Verification items for the finished model (mm, model axes). Face numbers are marked on the shaded views. Coordinates: 2 decimals unless noted, no trailing zeros. Write each loop counter-clockwise with the first axis right and the second up, starting at its lowest first coordinate (ties: lowest second). Pieces come first, ordered by that corner, then holes.
```python
from build123d import *

# Parameters (mm, degrees)
BOSS_EXTRUDE1_DEPTH = 25.5
SKETCH2_R           = 1.7
CUT_EXTRUDE1_DEPTH  = 31.42466105
FILLET1_R           = 3
SKETCH4_R           = 2.85
CUT_EXTRUDE2_DEPTH  = 30.815096847


with BuildPart() as part:
    # Sketch1 → Boss-Extrude1 (new body)
    with BuildSketch(Plane(origin=(0, 0, 0), x_dir=(0, 0, -1), z_dir=(1, 0, 0))):
        with BuildLine():
            Line((4.080441153, -0.4), (15, -0.4))
            Line((15, -0.4), (15, -3.4))
            Line((15, -3.4), (6.232976817, -3.4))
            ThreePointArc((6.232976817, -3.4), (0, -7.1), (-6.232976817, -3.4))
            Line((-6.232976817, -3.4), (-15, -3.4))
            Line((-15, -3.4), (-15, -0.4))
            Line((-15, -0.4), (-4.080441153, -0.4))
            ThreePointArc((-4.080441153, -0.4), (0, -4.1), (4.080441153, -0.4))
        make_face()
    extrude(amount=-BOSS_EXTRUDE1_DEPTH)

    # Sketch2 → Cut-Extrude1 (cut, through all)
    with BuildSketch(Plane(origin=(0, 0, 0), x_dir=(1, 0, 0), z_dir=(0, 1, 0))):
        with Locations(Location((-6, -10, 0), (0, 0, 270))):
            Circle(SKETCH2_R)
        with Locations(Location((-18, -10, 0), (0, 0, 270))):
            Circle(SKETCH2_R)
        with Locations(Location((-6, 10, 0), (0, 0, 270))):
            Circle(SKETCH2_R)
        with Locations(Location((-18, 10, 0), (0, 0, 270))):
            Circle(SKETCH2_R)
    extrude(amount=-CUT_EXTRUDE1_DEPTH, mode=Mode.SUBTRACT)

    # Fillet1
    fillet1_edges = [part.edges().sort_by_distance(p)[0] for p in [
        (0, -1.9, -15),
        (-12.75, -3.4, -6.232976817),
        (-25.5, -1.9, -15),
        (-25.5, -1.9, 15),
        (-12.75, -3.4, 6.232976817),
        (0, -1.9, 15),
    ]]
    fillet(fillet1_edges, radius=FILLET1_R)

    # Sketch4 → Cut-Extrude2 (cut, through all)
    with BuildSketch(Plane.XZ.offset(3.4)):
        with Locations((-18, -10)):
            Circle(SKETCH4_R)
        with Locations((-18, 10)):
            Circle(SKETCH4_R)
        with Locations((-6, 10)):
            Circle(SKETCH4_R)
        with Locations((-6, -10)):
            Circle(SKETCH4_R)
    extrude(amount=CUT_EXTRUDE2_DEPTH, mode=Mode.SUBTRACT)


solid = part.part
```
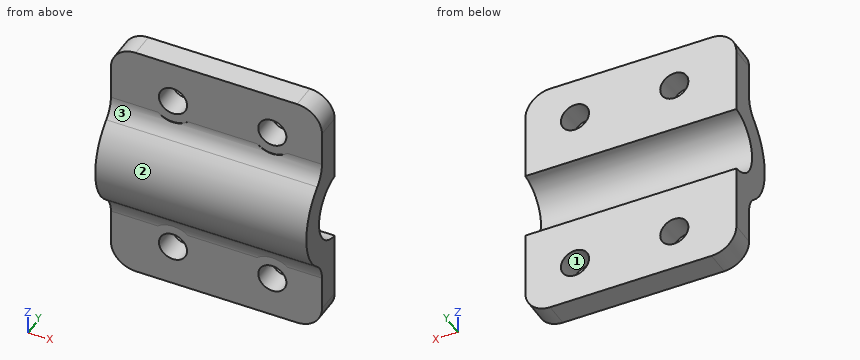
1. Gauge pin test, flat ends, axial feed: P1, Ø4, axis at x = -6, z = 10, coming from the -Y side; P2, Ø3, axis at x = -18, z = -10, coming from the +Y side; P3, Ø8.5, axis at x = -15.5, z = -10, coming from the -Y side. Record the tip position at first contact, or that the pin passes through.
2. Sectioned sample at C-C, the plane y = -1.25. Record the boundary of the cut face in (x, z).
3. Sectioned sample at B-B, the plane z = -10. Record the boundary of the cut face in (x, y), and give its area (3 significant figures).
4. Sectioned sample at A-A, the plane x = -6. Record the boundary of the cut face in (y, z), and give its area (3 significant figures).
5. Draft check along Z on the marked faces 1, 2 and 3. Enter one of: pulls with the +Z half, pulls with the -Z half, needs draft (parallel to the pull), parting line crosses it, or undercut.
6. Material ranges on L1, parallel to X at y = -1, z = -10; L2, parallel to Z at x = -4, y = -1.5; L3, parallel to Y at x = -8.5, z = -10.25, recorded low to high.
7. Sectioned sample at D-D, the plane x = -15. Record the boundary of the cut face in (y, z).
Outcome:
1. P1: stops at y = -3.4
1. P2: passes through
1. P3: stops at y = -4.22
2. outline: (-25.5, -12) arc R3 ccw to (-22.5, -15) - (-3, -15) arc R3 ccw to (0, -12) - (0, -3.9) - (-25.5, -3.9) - close; (-25.5, 3.9) - (0, 3.9) - (0, 12) arc R3 ccw to (-3, 15) - (-22.5, 15) arc R3 ccw to (-25.5, 12) - close; hole circle Ø3.4 at (-18, -10); hole circle Ø3.4 at (-18, 10); hole circle Ø3.4 at (-6, -10); hole circle Ø3.4 at (-6, 10)
3. outline: (-25.5, -3.4) - (-19.7, -3.4) - (-19.7, -0.4) - (-25.5, -0.4) - close; (-16.3, -3.4) - (-7.7, -3.4) - (-7.7, -0.4) - (-16.3, -0.4) - close; (-4.3, -3.4) - (0, -3.4) - (0, -0.4) - (-4.3, -0.4) - close
3. area: 56.1 mm2
4. outline: (-4.5, -5.49) arc R3 cw to (-3.47, -7.15) - (-3.4, -7.15) - (-3.4, -8.3) - (-0.4, -8.3) - (-0.4, -4.08) arc R4.1 cw to (-0.4, 4.08) - (-0.4, 8.3) - (-3.4, 8.3) - (-3.4, 7.15) - (-3.47, 7.15) arc R3 cw to (-4.5, 5.49) arc R7.1 ccw to start; (-3.4, -15) - (-0.4, -15) - (-0.4, -11.7) - (-3.4, -11.7) - close; (-3.4, 11.7) - (-0.4, 11.7) - (-0.4, 15) - (-3.4, 15) - close
4. area: 79.9 mm2
5. face 1: undercut
5. face 2: parting line crosses it
5. face 3: pulls with the +Z half
6. L1: x = -25.5 to -19.7, -16.3 to -7.7, -4.3 to 0
6. L2: z = -15 to -3.82, 3.82 to 15
6. L3: y = -3.4 to -0.4
7. outline: (-4.5, -5.49) arc R3 cw to (-3.4, -7.81) - (-3.4, -15) - (-0.4, -15) - (-0.4, -4.08) arc R4.1 cw to (-0.4, 4.08) - (-0.4, 15) - (-3.4, 15) - (-3.4, 7.81) arc R3 cw to (-4.5, 5.49) arc R7.1 ccw to start
